Model file for the job. Use its own axes, mm. Face numbers are marked on the shaded views. Coordinates: 2 decimals unless noted, no trailing zeros. Order: outer loops, then holes, each group sorted by start corner. A loop starts at its lowest first (then second) coordinate and runs counter-clockwise, first axis right, second up. Notation, with made-up numbers: (-6, 48.5) - (24, 48.5) arc R38 cw to (24, 86.5) - close; hole circle Ø9 at (-7.5, 38). An arc over 180 degrees is marked (long way). Put each result on its own line as item: value. Start each with the question number.
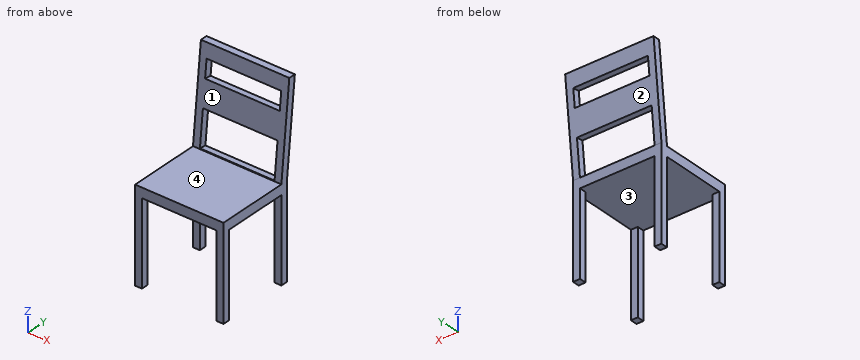
```python
from build123d import *

# Parameters (mm, degrees)
F0_W     = 450
F0_H     = 450
F1_DEPTH = 950
F2_W     = 50
F2_H     = 50
F2_W_2   = 330
F2_H_2   = 425
F3_DEPTH = 450.001
F4_W     = 380
F4_H     = 425
F5_DEPTH = 450.001
F6_W     = 380
F6_H     = 180
F6_H_2   = 90
F7_DEPTH = 447.528454


with BuildPart() as f1:
    # F0 (on Top) → F1 (new body)
    with BuildSketch(Plane.XY):
        Rectangle(F0_W, F0_H)
    extrude(amount=F1_DEPTH)

    # F2 (on face) → F3 (cut, through all)
    with BuildSketch(Plane.YZ.offset(225)):
        with Locations((200, 450)):
            Rectangle(F2_W, F2_H)
        Polygon((-225, 475), (140, 475), (190, 950), (-225, 950), align=None)
        with Locations((-25, 212.5)):
            Rectangle(F2_W_2, F2_H_2)
        with Locations((200, 212.5)):
            Rectangle(F2_W, F2_H_2)
        Polygon((175, 475), (225, 475), (225, 950), align=None)
    extrude(amount=-F3_DEPTH, mode=Mode.SUBTRACT)

    # F4 (on face) → F5 (cut, through all)
    with BuildSketch(Plane.XZ.offset(225)):
        with Locations((0, 212.5)):
            Rectangle(F4_W, F4_H)
    extrude(amount=-F5_DEPTH, mode=Mode.SUBTRACT)

    # F6 (on face) → F7 (cut, through all)
    with BuildSketch(Plane(origin=(0, 123.630137, -13.013699), x_dir=(-1, 0, 0), z_dir=(0, 0.994505, -0.104685))):
        with Locations((0, 580.709927)):
            Rectangle(F6_W, F6_H)
        with Locations((0, 848.334257)):
            Rectangle(F6_W, F6_H_2)
    extrude(amount=-F7_DEPTH, mode=Mode.SUBTRACT)


solid = f1.part
```
Item 1: Pull direction Y, two halves, no side cores. Call the marked faces 1, 2, 3 and 4: pulls with the +Y half, pulls with the -Y half, needs draft (parallel to the pull), parting line crosses it, or undercut.
Item 2: Wall check: line 1 along Y through (x, z) = (199.5, 68); line 2 along Z through (x, y) = (-100, 107); line 3 along Y through (x, z) = (-9, 460). Give the ranges that are in metal, low to high.
Item 3: Flat gauge pins, fed straight in: pin 1 Ø10.5 at (x, z) = (207, 216) entering from +Y; pin 2 Ø1 at (x, y) = (-120, 133.5) entering from -Z; pin 3 Ø1.5 at (x, y) = (-138.5, 35.5) entering from +Z. Where does each tip first touch, or does it go through?
Item 4: Slice it at C-C, the plane z = 77. Give the cut face in (x, y), plus the area to 3 significant figures.
Item 5: Slice it at D-D, the plane y = -77. Give the cut face in (x, z), plus the area to 3 significant figures.
Item 6: Slice it at B-B, the plane z = 819. Give the cut face in (x, y), plus the area to 3 significant figures.
Item 7: Slice it at A-A, the plane x = -71. Give the cut face in (y, z).
Here are the results:
1. face 1: pulls with the -Y half
1. face 2: pulls with the +Y half
1. face 3: undercut
1. face 4: needs draft
2. line 1: y = -225 to -190, 140 to 175
2. line 2: z = 425 to 475
2. line 3: y = -225 to 175
3. pin 1: stops at y = 175
3. pin 2: stops at z = 425
3. pin 3: stops at z = 475
4. outline: (-225, -225) - (-190, -225) - (-190, -190) - (-225, -190) - close; (-225, 140) - (-190, 140) - (-190, 175) - (-225, 175) - close; (190, -225) - (225, -225) - (225, -190) - (190, -190) - close; (190, 140) - (225, 140) - (225, 175) - (190, 175) - close
4. area: 4,900 mm^2
5. outline: (-225, 425) - (225, 425) - (225, 475) - (-225, 475) - close
5. area: 22,500 mm^2
6. outline: (-225, 176.21) - (-190, 176.21) - (-190, 211.21) - (-225, 211.21) - close; (190, 176.21) - (225, 176.21) - (225, 211.21) - (190, 211.21) - close
6. area: 2,450 mm^2
7. outline: (-225, 425) - (175, 425) - (175, 475) - (140.38, 478.64) - (140, 475) - (-225, 475) - close; (159.23, 657.65) - (193.84, 654.01) - (207.73, 785.91) - (173.11, 789.55) - close; (182.53, 879.06) - (217.15, 875.41) - (225, 950) - (190, 950) - close
